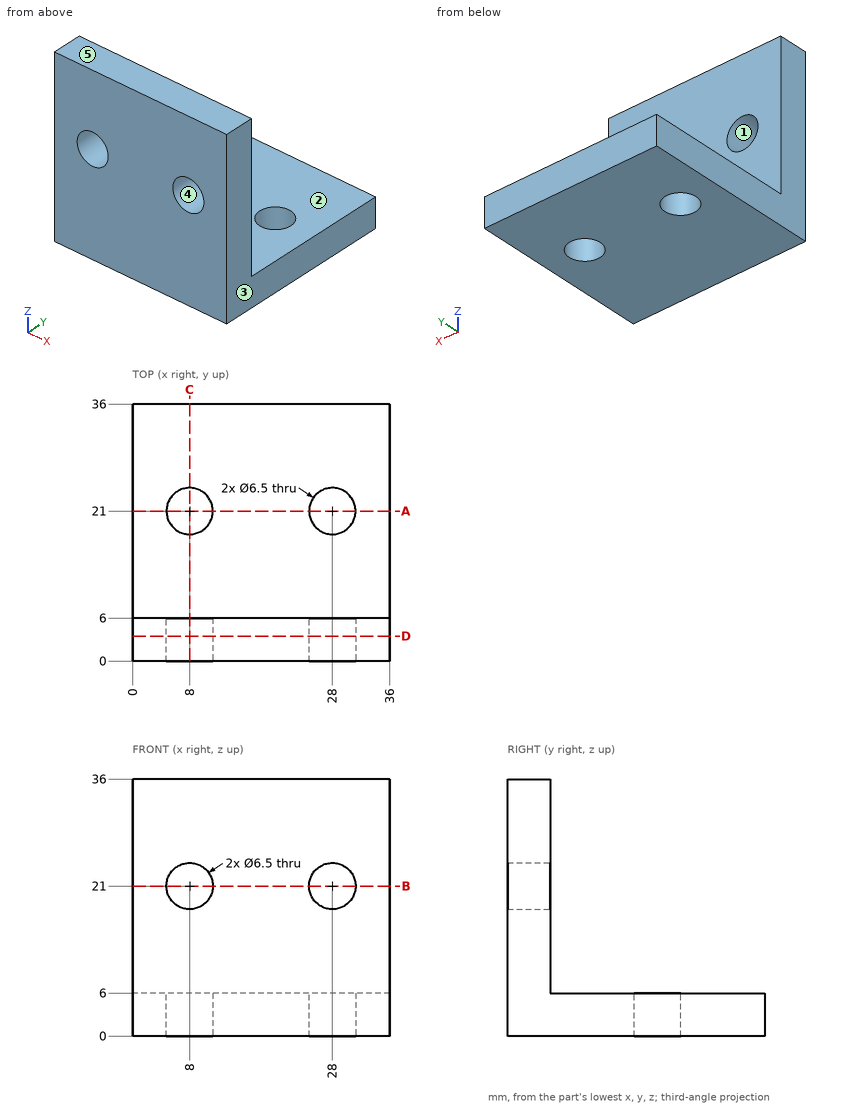
Can you work these out from the drawing? Everything is in mm from the part's minimum corner. A direction names the side the tool comes from. Round coordinates to 2 decimals unless told otherwise and drop trailing zeros. Write each loop counter-clockwise with the first axis right and the second up, starting at its lowest first coordinate (ties: lowest second). Pieces come first, ordered by that corner, then holes.
1. Suppose I cut it at C-C (x = 8). List the corners of the cut face in (y, z) for me.
2. I need wall thicknesses on L1, parallel to X at y = 1.35, z = 21; L2, parallel to Y at x = 28, z = 1.95. Which ranges of each line are inside material? Lowest first, please.
3. Suppose I cut it at D-D (y = 3.5). List the corners of the cut face in (x, z) for me, and give its area (3 significant figures).
4. If we mould it in two halves opening along X, with no side actions, what happens to the marked faces 3, 4 and 5? For each: released by +X, released by -X, zero draft, split by the parting line, or undercut.
5. Suppose I cut it at A-A (y = 21). List the corners of the cut face in (x, z) for me, and give its area (3 significant figures).
6. For the marked faces 1 and 2, which set-ups out of +Z, -Z, +X, -X, +Y, -Y let a thin tool reach every point of the face, with its end or its side?
7. Will these pins go through, and if not, where does the flat tip stop? pin 1 Ø3 at (x, y) = (16.5, 12) entering from -Z; pin 2 Ø9 at (x, y) = (23, 23) entering from +Z.
Answer sheet:
1. outline: (0, 0) - (17.75, 0) - (17.75, 6) - (6, 6) - (6, 17.75) - (0, 17.75) - close; (0, 24.25) - (6, 24.25) - (6, 36) - (0, 36) - close; (24.25, 0) - (36, 0) - (36, 6) - (24.25, 6) - close
2. L1: x = 0 to 4.75, 11.25 to 24.75, 31.25 to 36
2. L2: y = 0 to 17.75, 24.25 to 36
3. outline: (0, 0) - (36, 0) - (36, 36) - (0, 36) - close; hole circle Ø6.5 at (8, 21); hole circle Ø6.5 at (28, 21)
3. area: 1,230 mm2
4. face 3: released by +X
4. face 4: undercut
4. face 5: zero draft
5. outline: (0, 0) - (4.75, 0) - (4.75, 6) - (0, 6) - close; (11.25, 0) - (24.75, 0) - (24.75, 6) - (11.25, 6) - close; (31.25, 0) - (36, 0) - (36, 6) - (31.25, 6) - close
5. area: 138 mm2
6. face 1: +Y, -Y
6. face 2: +Z, +X, -X, +Y
7. pin 1: stops at z = 0
7. pin 2: stops at z = 6
